```python
from build123d import *

# Parameters (mm, degrees)
SKETCH006_R   = 1
SKETCH006_R_2 = 1.2
SKETCH006_R_3 = 1.491082
PAD002_DEPTH  = 1.6
SKETCH033_W   = 5.831177
SKETCH033_H   = 20.949042
PAD019_DEPTH  = 5.5
PAD021_DEPTH  = 2
SKETCH053_W   = 19.104945
SKETCH053_H   = 22.868039
PAD026_DEPTH  = 2
SKETCH058_W   = 43.228985
SKETCH058_H   = 5.789597
PAD028_DEPTH  = 4.3
SKETCH110_W   = 3.54
SKETCH110_H   = 12.73
PAD057_DEPTH  = 3
FILLET018_R   = 1.7


with BuildPart() as part:
    # Sketch006 → Pad002 (new body)
    with BuildSketch(Plane.XY.offset(3)):
        Polygon((30.75, 54.68), (30.75, -28.32), (28.95, -38.82), (26.75, -43.82), (19.75, -43.82), (19.75, -47.52), (-19.75, -47.52), (-19.75, -43.82), (-26.75, -43.82), (-28.95, -38.82), (-30.75, -28.32), (-30.75, 54.68), (-26.5, 54.68), (-26.5, 57.68), (26.5, 57.68), (26.5, 54.68), align=None)
        with Locations((-27.25, -32.12)):
            Circle(SKETCH006_R, mode=Mode.SUBTRACT)
        with Locations((15.75, -32)):
            Circle(SKETCH006_R, mode=Mode.SUBTRACT)
        with Locations((29.1, 50.68)):
            Circle(SKETCH006_R, mode=Mode.SUBTRACT)
        with Locations((-29.1, 50.68)):
            Circle(SKETCH006_R, mode=Mode.SUBTRACT)
        with Locations((-29.1, 5)):
            Circle(SKETCH006_R, mode=Mode.SUBTRACT)
        with Locations((-29.3, 13)):
            Circle(SKETCH006_R_2, mode=Mode.SUBTRACT)
        with Locations((29.3, 13)):
            Circle(SKETCH006_R_2, mode=Mode.SUBTRACT)
        with Locations((29.1, 5)):
            Circle(SKETCH006_R, mode=Mode.SUBTRACT)
        with Locations((-7.25, -45.92)):
            Circle(SKETCH006_R, mode=Mode.SUBTRACT)
        with Locations((-29.1, -25)):
            Circle(SKETCH006_R, mode=Mode.SUBTRACT)
        with Locations((29.1, -25)):
            Circle(SKETCH006_R, mode=Mode.SUBTRACT)
        with Locations((-14.007447, 49.274082)):
            Circle(SKETCH006_R_3, mode=Mode.SUBTRACT)
    extrude(amount=-PAD002_DEPTH)

    # Sketch033 (on Face30 of Pad002) → Pad019 (join)
    with BuildSketch(Plane(origin=(0, 0, 1.4), x_dir=(1, 0, 0), z_dir=(0, 0, -1))):
        with Locations((-22.462421, -27.118268)):
            Rectangle(SKETCH033_W, SKETCH033_H)
    extrude(amount=PAD019_DEPTH)

    # Sketch046 (on Face5 of Pad019) → Pad021 (join)
    with BuildSketch(Plane(origin=(0, 0, 1.4), x_dir=(1, 0, 0), z_dir=(0, 0, -1))):
        Polygon((21.00816, -56.937296), (21.00816, -41.937296), (6.00816, -41.937296), (6.00816, -56.937296), (6.00816, -59.937296), (17.00816, -59.937296), (17.00816, -56.937296), align=None)
    extrude(amount=PAD021_DEPTH)

    # Sketch053 (on Face5 of Pad021) → Pad026 (join)
    with BuildSketch(Plane(origin=(0, 0, 1.4), x_dir=(1, 0, 0), z_dir=(0, 0, -1))):
        with Locations((0.746086, -5.026741)):
            Rectangle(SKETCH053_W, SKETCH053_H)
    extrude(amount=PAD026_DEPTH)

    # Sketch058 (on Face4 of Pad026) → Pad028 (join)
    with BuildSketch(Plane.XY.offset(3)):
        with Locations((-0.757428, -40.205624)):
            Rectangle(SKETCH058_W, SKETCH058_H)
    extrude(amount=PAD028_DEPTH)

    # Sketch110 (on Face5 of Pad028) → Pad057 (join)
    with BuildSketch(Plane(origin=(0, 0, 1.4), x_dir=(1, 0, 0), z_dir=(0, 0, -1))):
        with Locations((20.398529, -31.503779)):
            Rectangle(SKETCH110_W, SKETCH110_H)
    extrude(amount=PAD057_DEPTH)

    # Fillet018
    fillet018_edges = [part.edges().sort_by_distance(p)[0] for p in [
        (18.628529, 25.138779, -0.1),
        (22.168529, 25.138779, -0.1),
        (22.168529, 37.868779, -0.1),
        (18.628529, 37.868779, -0.1),
    ]]
    fillet(fillet018_edges, radius=FILLET018_R)


solid = part.part
```
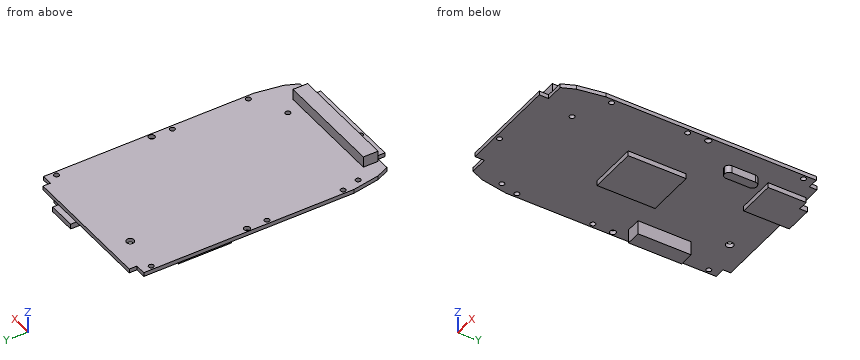
Could you check a few things on this model? Use its own coordinates, in mm. Round coordinates to 2 decimals unless told otherwise and drop trailing zeros. Loops run counter-clockwise (first coordinate to the right, second up) from the corner with the lowest first, then second, coordinate; pieces in that order, holes last.
Q1. Please list where these lines run through material, in increasing order: L1, parallel to Y at x = 15.75, z = 2; L2, parallel to X at y = 32.5, z = -0.75; L3, parallel to Z at x = -26, y = -18.5.
Q2. I want a section at C-C (y = -5). Write out the boundary of the cut face in (x, z), and give its area (3 significant figures).
Q3. I want a section at A-A (y = -25). Write out the boundary of the cut face in (x, z).
Q4. I want a section at B-B (x = 3.5). Write out the boundary of the cut face in (y, z), and give its area (3 significant figures).
Q5. For P1, Ø1.5, axis at x = 10.5, z = -1.5, coming from the +Y side; P2, Ø2, axis at x = -3, z = 1, coming from the +Y side; P3, Ø3, axis at x = 29.1, y = 50.68, coming from the -Z side; P4, Ø1.5, axis at x = 11, y = -28, coming from the +Z side, each with a flat end and sliding along its axis, tell me the tip position at first contact or that it passes through.
Answer below:
1. L1: y = -47.52 to -33, -31 to 57.68
1. L2: x = -25.38 to -19.55, 18.63 to 22.17
1. L3: z = 1.4 to 3
2. outline: (-30.75, 1.4) - (-8.81, 1.4) - (-8.81, -0.6) - (10.3, -0.6) - (10.3, 1.4) - (30.75, 1.4) - (30.75, 3) - (-30.75, 3) - close
2. area: 137 mm2
3. outline: (-30.75, 1.4) - (-30.1, 1.4) - (-30.1, 3) - (-30.75, 3) - close; (-28.1, 1.4) - (28.1, 1.4) - (28.1, 3) - (-28.1, 3) - close; (30.1, 1.4) - (30.75, 1.4) - (30.75, 3) - (30.1, 3) - close
4. outline: (-47.52, 1.4) - (-6.41, 1.4) - (-6.41, -0.6) - (16.46, -0.6) - (16.46, 1.4) - (57.68, 1.4) - (57.68, 3) - (-37.31, 3) - (-37.31, 7.3) - (-43.1, 7.3) - (-43.1, 3) - (-47.52, 3) - close
4. area: 239 mm2
5. P1: passes through
5. P2: stops at y = 57.68
5. P3: stops at z = 1.4
5. P4: stops at z = 3
